from build123d import *

# Parameters (mm, degrees)
SKETCH1_R               = 3
EXTRUDE1_DEPTH          = 22
SKETCH6_R               = 5
EXTRUDE2_DEPTH          = 6
CUT_EXTRUDE1_DEPTH      = 3.75
CHAMFER1_SIZE           = 0.3
CUT_EXTRUDE4_DEPTH      = 29.879058156
CUT_EXTRUDE4_DEPTH_BACK = 29.879058156
SKETCH13_R              = 0.79375


with BuildPart() as part:
    # Sketch1 → Extrude1 (new body)
    with BuildSketch(Plane.XY):
        Circle(SKETCH1_R)
    extrude(amount=-EXTRUDE1_DEPTH)

    # Sketch4 → Cut-Revolve1 (revolve, cut)
    with BuildSketch(Plane(origin=(0, 0, 0), x_dir=(0, 0, -1), z_dir=(1, 0, 0)), mode=Mode.PRIVATE) as cut_revolve1_sk:
        Polygon((0.632650852, 3), (0, 2.096480947), (0, 3), align=None)
    revolve(cut_revolve1_sk.sketch.rotate(Axis((0, 0, 0), (0, 0, -1)), 90), axis=Axis((0, 0, 0), (0, 0, -1)), mode=Mode.SUBTRACT)

    # Sketch6 → Extrude2 (add)
    with BuildSketch(Plane(origin=(0, 0, -22), x_dir=(-1, 0, 0), z_dir=(0, 0, -1))):
        Circle(SKETCH6_R)
    extrude(amount=EXTRUDE2_DEPTH)

    # Sketch7 → Cut-Extrude1 (cut)
    with BuildSketch(Plane(origin=(0, 0, -28), x_dir=(-1, 0, 0), z_dir=(0, 0, -1))):
        Polygon((0, 2.886751346), (-2.5, 1.443375673), (-2.5, -1.443375673), (0, -2.886751346), (2.5, -1.443375673), (2.5, 1.443375673), align=None)
    extrude(amount=-CUT_EXTRUDE1_DEPTH, mode=Mode.SUBTRACT)

    # Cut-Extrude2 cone 1 section (on through the dimple's axis) → Cut-Extrude2 (revolve, cut)
    with BuildSketch(Plane(origin=(0, 0, -28), x_dir=(0, 1, 0), z_dir=(1, 0, 0))):
        Polygon((0, 0), (2.886751346, 0), (0, 2.886751346), align=None)
    revolve(axis=Axis((0, 0, -28), (0, 0, 1)), mode=Mode.SUBTRACT)

    # Chamfer1
    chamfer1_edges = [part.edges().sort_by_distance(p)[0] for p in [
        (5, 0, -22),
        (5, 0, -28),
    ]]
    chamfer(chamfer1_edges, length=CHAMFER1_SIZE)

    # Sketch10 → Revolve1 (revolve)
    with BuildSketch(Plane(origin=(0, 0, 0), x_dir=(0, 0, -1), z_dir=(1, 0, 0))):
        Polygon((22, 3), (22, 0), (20.507359313, 0), (21.75, 3), align=None)
    revolve(axis=Axis((0, 0, -22), (0, 0, 1)))

    # Sketch13 → Cut-Extrude4 (cut, two sides: drawn at the far end of the back side and taken through both)
    with BuildSketch(Plane(origin=(0, 0, 0), x_dir=(0, 0, -1), z_dir=(1, 0, 0)).offset(-CUT_EXTRUDE4_DEPTH_BACK)):
        with Locations(Location((26.125, 0, 0), (0, 0, 180))):
            Circle(SKETCH13_R)
    extrude(amount=CUT_EXTRUDE4_DEPTH + CUT_EXTRUDE4_DEPTH_BACK, mode=Mode.SUBTRACT)


solid = part.part
Geometry: final body of the model. Coordinates: model frame, mm. A direction names the side the tool comes from. Give positions to 0.01 mm unless a question says otherwise; leave off trailing zeros. Loops run counter-clockwise (first coordinate to the right, second up) from the corner with the lowest first, then second, coordinate; pieces in that order, holes last. Notation, with made-up numbers: M 68,70.25 L 115,70.25 A24 cw 115,95.25 Z; hole C -11.75,-6.75 d3. An arc over 180 degrees is marked long. Put each result on its own line as item: value. Start each with the question number.
1) Cut plane B-B (z = -15). Output: boundary loops of the cut face in (x, y).
2) Ray query, line 1 along Z through (x, y) = (-3.75, -2.5); line 2 along Z through (x, y) = (1.25, 0.25); line 3 along Y through (x, z) = (0, -1). Return the intervals inside material, ascending.
3) Pull-direction query (Y, two-part tool) for faces 1 (the cylindrical face through (-3, 0, -11)), 2 (the flat face through (-1.233, -2.175, -26.151)), 3 (the flat face through (0, 0, 0)); classes: pulls with the +Y half, pulls with the -Y half, needs draft (parallel to the pull), parting line crosses it, or undercut.
4) Access query for faces 4 (the cylindrical face through (3.73, -0.24, -25.37)), 5 (the conical face through (1.328, -2.34, -27.804)), 6 (the flat face through (-1, -3, -22)). Directions: +Z, -Z, +X, -X, +Y, -Y. A direction counts if a zero-diameter tool reaches every point of the face in a straight line with its end or side. Return the directions, or none.
5) Contact query for flat-ended pins moving along their axis: pin 1 (1.5 mm diameter, centred on x = 4, y = 3.5, fed in from -Z); pin 2 (6 mm diameter, centred on x = -0.5, z = -17.5, fed in from -Y); pin 3 (1.5 mm diameter, centred on x = -1.5, y = 0.5, fed in from -Z); pin 4 (1 mm diameter, centred on x = 2.5, y = 1, fed in from +Z). Output: stop coordinate, or through.
6) Cut plane A-A (y = 0). Output: boundary loops of the cut face in (x, z).
Verdict:
1. outline: C 0,0 d6
2. line 1: -28 to -22
2. line 2: -24.25 to 0
2. line 3: -3 to 3
3. face 1: parting line crosses it
3. face 2: undercut
3. face 3: needs draft
4. face 4: +X, -X
4. face 5: -Z
4. face 6: +Z
5. pin 1: z = -28
5. pin 2: y = -3
5. pin 3: z = -24.25
5. pin 4: z = -0.07
6. outline: M -5,-27.7 L -4.7,-28 L -2.89,-28 L -2.5,-27.61 L -2.5,-26.92 L -5,-26.92 Z; M -5,-25.33 L -2.5,-25.33 L -2.5,-24.25 L 2.5,-24.25 L 2.5,-25.33 L 5,-25.33 L 5,-22.3 L 4.7,-22 L 3,-22 L 3,-0.63 L 2.1,0 L -2.1,0 L -3,-0.63 L -3,-22 L -4.7,-22 L -5,-22.3 Z; M 2.5,-27.61 L 2.89,-28 L 4.7,-28 L 5,-27.7 L 5,-26.92 L 2.5,-26.92 Z
